from build123d import *

# Parameters (mm, degrees)
ESQUISSE1_W                     = 10
ESQUISSE1_H                     = 10
BOSS_EXTRU_1_DEPTH              = 82.5
TROU_TARAUD_M3X0_52_D           = 2.5
TROU_TARAUD_M3X0_52_CSINK_D     = 3.05
TROU_TARAUD_M3X0_52_CSINK_ANGLE = 90


with BuildPart() as part:
    # Esquisse1 → Boss.-Extru.1 (new, symmetric)
    with BuildSketch(Plane.XY):
        Rectangle(ESQUISSE1_W, ESQUISSE1_H)
    extrude(amount=BOSS_EXTRU_1_DEPTH, both=True)

    # Trou taraudé M3x0.52 (through all)
    with Locations(Plane(origin=(0, 5, 0), x_dir=(1, 0, 0), z_dir=(0, 1, 0))):
        with Locations((0, 68), (0, -68)):
            CounterSinkHole(TROU_TARAUD_M3X0_52_D / 2, TROU_TARAUD_M3X0_52_CSINK_D / 2, counter_sink_angle=TROU_TARAUD_M3X0_52_CSINK_ANGLE)


solid = part.part
Verification items for the finished model (mm, model axes). Give positions to 0.01 mm unless a question says otherwise; leave off trailing zeros. Put each result on its own line as item: value. Start each with the question number.
1. Scan lines: line 1 along Z through (x, y) = (0, 2.75); line 2 along X through (y, z) = (0.5, 68); line 3 along Z through (x, y) = (1, -2.25). Record each from-to range of solid material in increasing order. Write a range as [from, to].
2. Draft check along X on faces 1 (the face through (5, 0, 1)), 2 (the face through (0, 0, -82.5)), 3 (the face through (0.16, -0.21, -69.24)). Enter one of: +X half, -X half, draft (parallel to the pull), parting line (faces both ways), or undercut.
3. Go/stop test with a flat-tipped pin: pin 1 Ø2 at (x, z) = (0, 68) entering from +Y. Record where the tip stops, or that it passes through.
Answer list:
1. line 1: [-82.5, -69.25], [-66.75, 66.75], [69.25, 82.5]
1. line 2: [-5, -1.25], [1.25, 5]
1. line 3: [-82.5, -68.75], [-67.25, 67.25], [68.75, 82.5]
2. face 1: +X half
2. face 2: draft
2. face 3: undercut
3. pin 1: through
